```python
from build123d import *

# Parameters (mm, degrees)
F_6_CLEARANCE_HOLE1_D     = 3.7973
BOSS_EXTRUDE1_START       = 10
SKETCH4_R                 = 1.25
BOSS_EXTRUDE1_DEPTH       = 1.5
F_8_32_TAPPED_HOLE1_D     = 3.4544
F_8_32_TAPPED_HOLE1_DEPTH = 10.708
F_8_32_TAPPED_HOLE1_TIP   = 1.037806461
MOVE_FACE1_BY             = 6.55
CHAMFER1_SIZE             = 0.3


with BuildPart() as part:
    # Sketch1 → Revolve1 (revolve)
    with BuildSketch(Plane.XY, mode=Mode.PRIVATE) as revolve1_sk:
        Polygon((-9.5, 3), (2.5, 3), (2.5, 4), (0, 4), (0, 14.2621), (-2.5, 14.2621), (-2.5, 11.5), (-9.5, 11.5), align=None)
    revolve(revolve1_sk.sketch.rotate(Axis((0, 0, 0), (1, 0, 0)), 90), axis=Axis((0, 0, 0), (1, 0, 0)))

    # 6 Clearance Hole1 (through all)
    with Locations(Plane(origin=(0, 0, 0), x_dir=(0, 0, -1), z_dir=(1, 0, 0))):
        with Locations((-8, 0), (0, 8), (0, -8), (8, 0)):
            Hole(F_6_CLEARANCE_HOLE1_D / 2)

    # Sketch4 → Boss-Extrude1 (add)
    with BuildSketch(Plane(origin=(0, 0, 0), x_dir=(-1, 0, 0), z_dir=(0, 0.7071067811865464, 0.7071067811865488)).offset(BOSS_EXTRUDE1_START)):
        with Locations((6, 0)):
            Circle(SKETCH4_R)
    extrude(amount=BOSS_EXTRUDE1_DEPTH)

    # 8-32 Tapped Hole1
    with Locations(Plane(origin=(0, 8.131727984, 8.131727984), x_dir=(1, 0, 0), z_dir=(0, 0.7071067811865465, 0.7071067811865487))):
        with Locations((-6, 0)):
            Hole(F_8_32_TAPPED_HOLE1_D / 2, depth=F_8_32_TAPPED_HOLE1_DEPTH)
            with Locations((0, 0, -(F_8_32_TAPPED_HOLE1_DEPTH + F_8_32_TAPPED_HOLE1_TIP / 2))):  # 118° drill point
                Cone(0, F_8_32_TAPPED_HOLE1_D / 2, F_8_32_TAPPED_HOLE1_TIP, mode=Mode.SUBTRACT)

    # Move Face1: a face moved outward by 6.55
    extrude(part.faces().sort_by_distance((2.5, 3.2, 0))[0], amount=MOVE_FACE1_BY, dir=(1, 0, 0))

    # Chamfer1
    chamfer1_edges = [part.edges().sort_by_distance(p)[0] for p in [
        (-9.5, 0, -3),
        (9.05, 0, -3),
        (9.05, 0, -4),
        (0, 0, -14.2621),
        (-2.5, 0, -14.2621),
        (-9.5, 0, -11.5),
    ]]
    chamfer(chamfer1_edges, length=CHAMFER1_SIZE)


solid = part.part
```
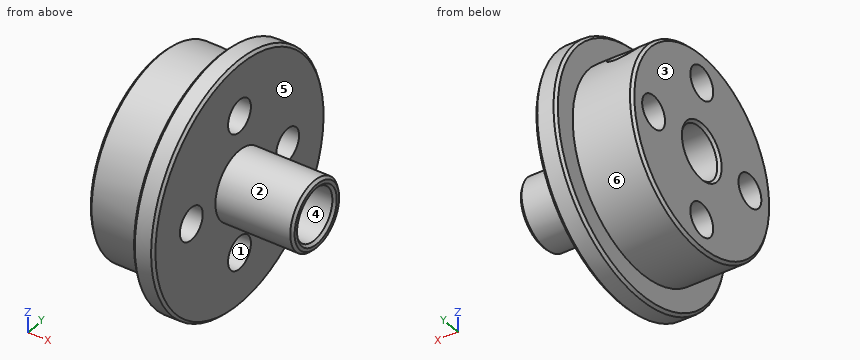
Could you check a few things on this model? Use its own coordinates, in mm. Face numbers are marked on the shaded views. A direction names the side the tool comes from. Coordinates: 2 decimals unless noted, no trailing zeros. Write each loop counter-clockwise with the first axis right and the second up, starting at its lowest first coordinate (ties: lowest second). Pieces come first, ordered by that corner, then holes. Notation, with made-up numbers: (22.25, -16) -> (26.25, -16) arc R25 cw to (26.25, 12) -> close; hole circle Ø6 at (35.5, 70.5). An arc over 180 degrees is marked (long way). One line per question, with ' | ' between items. Start each with the question number.
1. For the marked faces 4, 5 and 6, which set-ups out of +Z, -Z, +X, -X, +Y, -Y let a thin tool reach every point of the face, with its end or its side?
2. If we section it at A-A (y = 6.75): Count the separate pieces of the cut face and the enclosed holes in it, and give its area (3 significant figures).
3. If we section it at C-C (x = 4.25): Please give me the cut outline in (y, z).
4. If we section it at B-B (x = -6.25): Please give me the cut outline in (y, z) (3 decimals), and give its area (3 significant figures).
5. Thinking about a two-plate mould opening in Y: for the marked faces 1, 2 and 3, which applies, pulls with the +Y half, pulls with the -Y half, needs draft (parallel to the pull), parting line crosses it, or undercut?
6. Will these pins go through, and if not, where does the flat tip stop? P1, Ø4, axis at x = -7, z = 3.5, coming from the -Y side; P2, Ø2, axis at x = -5, y = 7.5, coming from the -Z side; P3, Ø3, axis at y = 0, z = 8, coming from the +X side; P4, Ø5, axis at x = -2.5, z = -5.5, coming from the -Y side.
7. Please list where these lines run through material, in increasing order: line 1 along Y through (x, z) = (-6.75, 0); line 2 along X through (y, z) = (1.75, 4.5); line 3 along Y through (x, z) = (-2.25, 0).
Return value:
1) face 4: +X, -X | face 5: +X | face 6: -X
2) separate pieces: 2 | enclosed holes: 1 | area: 152 mm²
3) outline: circle Ø8 at (0, 0); hole circle Ø6 at (0, 0)
4) outline: (0.535, 2.952) -> (6.833, 9.25) arc R11.5 ccw (long way) to (9.25, 6.833) -> (2.952, 0.535) arc R3 cw (long way) to start; hole circle Ø3.797 at (-8, 0); hole circle Ø3.797 at (0, -8); hole circle Ø3.797 at (0, 8); hole circle Ø3.797 at (8, 0) | area: 312 mm²
5) face 1: undercut | face 2: parting line crosses it | face 3: needs draft
6) P1: stops at y = -11.4 | P2: stops at z = -9.49 | P3: passes through | P4: stops at y = -13.94
7) line 1: y = -11.5 to -9.9, -6.1 to -3, 3 to 6.1, 9.9 to 11.5 | line 2: x = -9.5 to 0 | line 3: y = -14.21 to -9.9, -6.1 to -3, 3 to 6.1, 9.9 to 14.21
